from build123d import *

# Parameters (mm, degrees)
ESQUISSE1_R             = 4.125
ESQUISSE1_R_2           = 2.125
BOSS_EXTRU_1_DEPTH      = 2
BOSS_EXTRU_2_START      = -2
BOSS_EXTRU_2_DEPTH      = 2
ENL_V_MAT_EXTRU_1_DEPTH = 48.690657123
BOSS_EXTRU_3_START      = -2
BOSS_EXTRU_3_DEPTH      = 2
CONG_1_R                = 1
CONG_2_R                = 2


with BuildPart() as part:
    # Esquisse1 → Boss.-Extru.1 (new body)
    with BuildSketch(Plane.XY):
        with Locations(Location((22.625964543, -8.5, 0), (0, 0, 270))):
            Circle(ESQUISSE1_R)
        with Locations(Location((22.625964543, -8.5, 0), (0, 0, 270))):
            Circle(ESQUISSE1_R_2, mode=Mode.SUBTRACT)
    extrude(amount=BOSS_EXTRU_1_DEPTH)

    # Esquisse2 → Boss.-Extru.2 (add)
    with BuildSketch(Plane.XY.offset(2).offset(BOSS_EXTRU_2_START)):
        with BuildLine():
            Line((30.509764166, -23.030033129), (25.42611418, -23.030033129))
            Line((25.42611418, -23.030033129), (18.953657758, -10.378772971))
            ThreePointArc((18.953657758, -10.378772971), (23.931920923, -12.412812663), (26.690529558, -7.796482951))
            Line((26.690529558, -7.796482951), (28.668432745, -19.223805295))
            Line((28.668432745, -19.223805295), (31.625964543, -19.223805295))
            ThreePointArc((31.625964543, -19.223805295), (38.131775725, -11.04447664), (37.160125022, -0.638570082))
            Line((37.160125022, -0.638570082), (39.798855089, 0.788701312))
            ThreePointArc((39.798855089, 0.788701312), (40.551713625, -13.225604632), (30.509764166, -23.030033129))
        make_face()
    extrude(amount=BOSS_EXTRU_2_DEPTH)

    # Esquisse3 → Enlèv. mat.-Extru.1 (cut, through all)
    with BuildSketch(Plane.XY.offset(2)):
        with BuildLine():
            ThreePointArc((38.167376486, -5.226235195), (36.438745559, -1.907826674), (35.54029783, -5.540014951))
            ThreePointArc((35.54029783, -5.540014951), (35.031758868, -6.882600454), (35.553780718, -8.220001253))
            ThreePointArc((35.553780718, -8.220001253), (34.75530459, -9.413141471), (34.961960594, -10.833859953))
            ThreePointArc((34.961960594, -10.833859953), (33.914765028, -11.815964406), (33.795387502, -13.246662387))
            ThreePointArc((33.795387502, -13.246662387), (32.553529245, -13.967034361), (32.114280515, -15.333858513))
            ThreePointArc((32.114280515, -15.333858513), (30.552699493, -18.734073905), (33.972916342, -17.21680112))
            ThreePointArc((33.972916342, -17.21680112), (35.668723842, -16.476130338), (36.031089318, -14.661454735))
            ThreePointArc((36.031089318, -14.661454735), (37.515935524, -13.55710514), (37.459320378, -11.707469768))
            ThreePointArc((37.459320378, -11.707469768), (38.656556802, -10.296448426), (38.183883536, -8.507332369))
            ThreePointArc((38.183883536, -8.507332369), (39.031708248, -6.862476892), (38.167376486, -5.226235195))
        make_face()
    extrude(amount=-ENL_V_MAT_EXTRU_1_DEPTH, mode=Mode.SUBTRACT)

    # Esquisse4 → Boss.-Extru.3 (add)
    with BuildSketch(Plane.XY.offset(2).offset(BOSS_EXTRU_3_START)):
        with BuildLine():
            Line((30.509764166, -23.030033129), (32.509764166, -23.030033129))
            ThreePointArc((32.509764166, -23.030033129), (41.131762211, -13.249116028), (40.289284919, -0.23775862))
            ThreePointArc((40.289284919, -0.23775862), (40.336178222, -13.75207443), (30.509764166, -23.030033129))
        make_face()
    extrude(amount=BOSS_EXTRU_3_DEPTH)

    # Congé1
    cong_1_edges = [part.edges().sort_by_distance(p)[0] for p in [
        (37.160125022, -0.638570082, 1),
    ]]
    fillet(cong_1_edges, radius=CONG_1_R)

    # Congé2
    cong_2_edges = [part.edges().sort_by_distance(p)[0] for p in [
        (28.668432745, -19.223805295, 1),
    ]]
    fillet(cong_2_edges, radius=CONG_2_R)


solid = part.part
Geometry: final body of the model. Coordinates: model frame, mm. A direction names the side the tool comes from. Round coordinates to 2 decimals unless told otherwise and drop trailing zeros. Write each loop counter-clockwise with the first axis right and the second up, starting at its lowest first coordinate (ties: lowest second). Pieces come first, ordered by that corner, then holes. Notation, with made-up numbers: M -30.75,33.5 L -10.75,33.5 A27 cw -10.75,56.5 Z; hole C 51,76 d5. An arc over 180 degrees is marked long. Write item = value, one per line.
Item 1: Section query C-C on x = 35.5. Return loops of the section in (y, z), then the cut area to 3 significant figures.
Findings:
outline = M -21.16,0 L -16.66,0 L -16.66,2 L -21.16,2 Z
area = 9.00 mm^2
Item 2: Material intervals for line 1 along X through (y, z) = (-8.5, 1.55); line 2 along X through (y, z) = (-10.25, 1); line 3 along Y through (x, z) = (22.5, 1.8), sorted ascending. Write a range as [from, to].
Findings:
line_1 = [18.5, 20.5], [24.75, 26.81], [38.64, 42.03]
line_2 = [18.89, 21.42], [23.83, 27.12], [38.67, 41.86]
line_3 = [-17.31, -10.62], [-6.38, -4.38]
Item 3: Access query for faces 4 (the face through (41.07, -13.43, 0.99)), 5 (the face through (37.867, -11.845, 0.986)), 6 (the face through (29, -18.7, 1)), 7 (the face through (37.73, -1.89, 0.99)). Directions: +Z, -Z, +X, -X, +Y, -Y. A direction counts if a zero-diameter tool reaches every point of the face in a straight line with its end or side. Return the directions, or none.
Findings:
face_4 = +Z, -Z, +X
face_5 = +Z, -Z
face_6 = +Z, -Z, +Y
face_7 = +Z, -Z, -X
Item 4: Pull-direction query (X, two-part tool) for faces 1 (the face through (21.333, -6.814, 0.986)), 2 (the face through (27.6, -15.5, 2)), 3 (the face through (40.049, 0.287, 0.986)); classes: pulls with the +X half, pulls with the -X half, needs draft (parallel to the pull), parting line crosses it, or undercut.
Findings:
face_1 = undercut
face_2 = needs draft
face_3 = pulls with the +X half
Item 5: Pin query (flat end, axial travel): P1, Ø0.5, axis at x = 31, z = 1, coming from the +Y side; P2, Ø1, axis at x = 23, y = -9, coming from the +Z side (3 decimals). Return the tip coordinate at first contact, or that it passes through.
Findings:
P1 = -19.22
P2 = through
Item 6: Section query A-A on y = -8.75. Return loops of the section in (x, z), then the cut area to 3 significant figures.
Findings:
outline = M 18.51,0 L 20.52,0 L 20.52,2 L 18.51,2 Z; M 24.74,0 L 26.86,0 L 26.86,2 L 24.74,2 Z; M 38.61,0 L 42.01,0 L 42.01,2 L 38.61,2 Z
area = 15.1 mm^2
